```python
from build123d import *

# Parameters (mm, degrees)
F0_R     = 46.938629
F1_DEPTH = 25.4
F2_W     = 70.104
F2_H     = 10.672496
F3_DEPTH = 12.7


with BuildPart() as f1:
    # F0 (on Front) → F1 (new body)
    with BuildSketch(Plane.XZ):
        Circle(F0_R)
    extrude(amount=F1_DEPTH)

    # F2 (on face) → F3 (cut, symmetric)
    with BuildSketch(Plane.XZ.offset(25.4)):
        with Locations((0.886691, 5.336248)):
            Rectangle(F2_W, F2_H)
    extrude(amount=F3_DEPTH, both=True, mode=Mode.SUBTRACT)


solid = f1.part
```
Source: CAD feature listing. Evaluate the final solid. Frame: model axes, mm. A direction names the side the tool comes from. Round coordinates to 2 decimals unless told otherwise and drop trailing zeros. Loops run counter-clockwise (first coordinate to the right, second up) from the corner with the lowest first, then second, coordinate; pieces in that order, holes last. Notation, with made-up numbers: (-16, 19.5) - (26, 19.5) arc R23 cw to (26, 33.5) - close; hole circle Ø2 at (1.5, 72). An arc over 180 degrees is marked (long way). Use CSV: the item, a comma, the result in double quotes.
Q1. Pin query (flat end, axial travel): pin 1 Ø3 at (y, z) = (-14.5, 15.5) entering from +X; pin 2 Ø11.5 at (y, z) = (-16, 7.5) entering from -X; pin 3 Ø3 at (x, y) = (-36, -14) entering from -Z. Return the tip coordinate at first contact, or that it passes through.
Reported:
pin 1,"x = 44.8"
pin 2,"x = -46.91"
pin 3,"z = -31.83"
Q2. Section query B-B, the plane x = 0. Output: boundary loops of the cut face in (y, z).
Reported:
outline,"(-25.4, -46.94) - (0, -46.94) - (0, 46.94) - (-25.4, 46.94) - (-25.4, 10.67) - (-12.7, 10.67) - (-12.7, 0) - (-25.4, 0) - close"
Q3. Section query D-D, the plane z = -14. Output: boundary loops of the cut face in (x, y), then the cut area to 3 significant figures.
Reported:
outline,"(-44.8, -25.4) - (44.8, -25.4) - (44.8, 0) - (-44.8, 0) - close"
area,"2,280 mm^2"
Q4. Reachability of faces 4 (the flat face through (-34.165, -19, 5)), 5 (the flat face through (-1, -25.4, -10)) from +Z, -Z, +X, -X, +Y, -Y: full face, straight path, thin tool, end or side. Return the list, or none.
Reported:
face 4,"-Y"
face 5,"+Z, -Z, +X, -X, -Y"
Q5. Section query C-C, the plane z = 3. Output: boundary loops of the cut face in (x, y).
Reported:
outline,"(-46.84, -25.4) - (-34.17, -25.4) - (-34.17, -12.7) - (35.94, -12.7) - (35.94, -25.4) - (46.84, -25.4) - (46.84, 0) - (-46.84, 0) - close"
Q6. Ray query, line 1 along Z through (x, y) = (1, -21.75); line 2 along X through (y, z) = (-19.5, -1); line 3 along Y through (x, z) = (-5, 2). Return the intervals inside material, ascending.
Reported:
line 1,"-46.93 to 0, 10.67 to 46.93"
line 2,"-46.93 to 46.93"
line 3,"-12.7 to 0"
Q7. Section query A-A, the plane y = -15. Output: boundary loops of the cut face in (x, z).
Reported:
outline,"circle Ø93.88 at (0, 0); hole (-34.17, 0) - (35.94, 0) - (35.94, 10.67) - (-34.17, 10.67) - close"
Q8. Mould query, pull axis X, two halves, no side actions, for faces 1 (the flat face through (0, -19, 0)), 2 (the flat face through (-1, 0, 1)), 3 (the cylindrical face through (-46.893, -12.522, 2.064)). Classes: pulls with the +X half, pulls with the -X half, needs draft (parallel to the pull), parting line crosses it, or undercut.
Reported:
face 1,"undercut"
face 2,"needs draft"
face 3,"parting line crosses it"
